Autodesk Inventor part; units mm, degrees
ref_plane "Work Plane1" through (0, 0, 5.75) normal (0, 0, 1) x (1, 0, 0)
ref_plane "YZ Plane" through (0, 0, 0) normal (1, 0, 0) x (0, 1, 0)
ref_plane "XZ Plane" through (0, 0, 0) normal (0, 1, 0) x (-1, 0, 0)
sketch "Sketch1" plane through (0, 0, 0) normal (0, 1, 0) x (-1, 0, 0)
  circle A0 centre (0, 0) radius 5.75
  dimension "d0" = 11.5
extrude "Extrusion1" add sketch "Sketch1" along normal blind 100
sketch "Sketch2" plane through (0, 100, 0) normal (0, 1, 0) x (1, 0, 0)
  circle A0 centre (0, 0) radius 16
  dimension "d3" = 32
extrude "Extrusion2" add sketch "Sketch2" along normal blind 5
sketch "Sketch3" plane through (0, 105, 0) normal (0, 1, 0) x (1, 0, 0)
  circle A0 centre (0, 0) radius 9
  dimension "d6" = 18
extrude "Extrusion3" cut sketch "Sketch3" against normal blind 1
ref_plane "Work Plane1" through (0, 0, 5.75) normal (0, 0, 1) x (1, 0, 0)
sketch "Sketch4" plane through (0, 0, 5.75) normal (0, 0, 1) x (1, 0, 0)
  line L0 (5.75, 100) -> (-5.75, 100)
  line L1 (5.75, 0) -> (-5.75, 0)
  line L2 (0, 0) -> (0, 5)
  circle A0 centre (0, 5) radius 1.5
  dimension "d9" = 5
  dimension "d10" = 3
extrude "Extrusion4" cut sketch "Sketch4" against normal blind 11.5
chamfer "Chamfer1" distance 1 angle 45 1 edges at (5.75, 0, 0)
sketch "Sketch5" plane through (0, 0, 0) normal (0, 0, 1) x (1, 0, 0)
  line L0 (0, 0) -> (0, 42.5)
  line L1 (0, 42.5) -> (0, 32.5)
  line L2 (0, 42.5) -> (0, 52.5)
  circle A0 centre (0, 52.5) radius 2.5
  dimension "d16" = 42.5
  dimension "d17" = 10
  dimension "d18" = 10
  dimension "d19" = 5
extrude "Extrusion5" cut sketch "Sketch5" along normal mid plane 13
sketch "Sketch7" plane through (0, 105, 0) normal (0, 1, 0) x (1, 0, 0)
  circle A0 centre (0, 0) radius 9
  line L0 (-9, 0) -> (-16, 0)
  circle A1 centre (0, 0) radius 16
  circle A2 centre (-12.5, 0) radius 1.55
  dimension "d22" = 3.1
extrude "Extrusion6" cut sketch "Sketch7" against normal up to surface (5 mm away) contours A2 L0 | L0 A2
chamfer "Chamfer2" distance 0.3 angle 45 1 edges at (-14.05, 100, 0)
chamfer "Chamfer3" distance 0.3 angle 45 2 edges at (-2.5, 52.5, 5.1781) (-2.5, 52.5, -5.1781)
properties part number "wał_hamulca" material "ABS Plastic"
Source: CAD feature listing. Evaluate the final solid. Frame: model axes, mm. A direction names the side the tool comes from. Round coordinates to 2 decimals unless told otherwise and drop trailing zeros. Order: outer loops, then holes, each group sorted by start corner. A loop starts at its lowest first (then second) coordinate and runs counter-clockwise, first axis right, second up. Notation, with made-up numbers: (23.25, 28.25) -> (69.25, 28.25) arc R27 ccw to (69.25, 50.25) -> close; hole circle Ø7 at (15.5, 43.5). An arc over 180 degrees is marked (long way). Use CSV: the item, a comma, the result in double quotes.
(1) First-contact query: pin 1 Ø5.5 at (x, z) = (-0.5, 3.5) entering from +Y; pin 2 Ø5 at (x, y) = (-5, 20.5) entering from +Z; pin 3 Ø12 at (x, z) = (-5, -5) entering from -Y; pin 4 Ø8 at (x, y) = (0, 52.5) entering from +Z. Flat tips, straight axial feed; report the tip coordinate or a pass-through.
Report:
pin 1,"y = 104"
pin 2,"z = 5.18"
pin 3,"y = 0"
pin 4,"z = 5.75"
(2) Section C-C on y = 5. Return the cut outline in (x, z).
Report:
outline,"(-1.5, -5.55) -> (-1.5, 5.55) arc R5.75 ccw to start; (1.5, -5.55) arc R5.75 ccw to (1.5, 5.55) -> close"
(3) Section D-D on y = 88. Return the cut outline in (x, z), and give its area (3 significant figures).
Report:
outline,"circle Ø11.5 at (0, 0)"
area,"104 mm^2"
(4) Section B-B on x = -12.5. Return the cut outline in (y, z).
Report:
outline,"(100, -9.99) -> (105, -9.99) -> (105, -1.55) -> (100.3, -1.55) -> (100, -1.85) -> close; (100, 1.85) -> (100.3, 1.55) -> (105, 1.55) -> (105, 9.99) -> (100, 9.99) -> close"
(5) Access query for faces 1 (the face through (7, 105, 7)), 2 (the face through (0, 104, 0)), 3 (the face through (7, 100, 0)). Directions: +Z, -Z, +X, -X, +Y, -Y. A direction counts if a zero-diameter tool reaches every point of the face in a straight line with its end or side. Return the directions, or none.
Report:
face 1,"+Z, -Z, +X, -X, +Y"
face 2,"+Y"
face 3,"-Y"
(6) Pull-direction query (Z, two-part tool) for faces 4 (the face through (-2.653, 49.807, 5.101)), 5 (the face through (0, 0, 0)), 6 (the face through (-13.73, 102.68, 0.94)); classes: +Z half, -Z half, draft (parallel to the pull), parting line (faces both ways), or undercut.
Report:
face 4,"parting line"
face 5,"draft"
face 6,"undercut"
(7) Ray query, L1, parallel to Y at x = 0, z = 1.25; L2, parallel to Z at x = 0, y = 104.35; L3, parallel to X at y = 104.3, z = 0. Return the intervals inside material, ascending.
Report:
L1,"0 to 3.5, 6.5 to 50, 55 to 104"
L2,"-16 to -9, 9 to 16"
L3,"-16 to -14.05, -10.95 to -9, 9 to 16"
(8) Section A-A on z = 0. Return the cut outline in (x, y), and give its area (3 significant figures).
Report:
outline,"(-16, 100) -> (-14.35, 100) -> (-14.05, 100.3) -> (-14.05, 105) -> (-16, 105) -> close; (-10.95, 100.3) -> (-10.65, 100) -> (-5.75, 100) -> (-5.75, 1) -> (-4.75, 0) -> (4.75, 0) -> (5.75, 1) -> (5.75, 100) -> (16, 100) -> (16, 105) -> (9, 105) -> (9, 104) -> (-9, 104) -> (-9, 105) -> (-10.95, 105) -> close; hole circle Ø5 at (0, 52.5); hole circle Ø3 at (0, 5)"
area,"1,250 mm^2"
